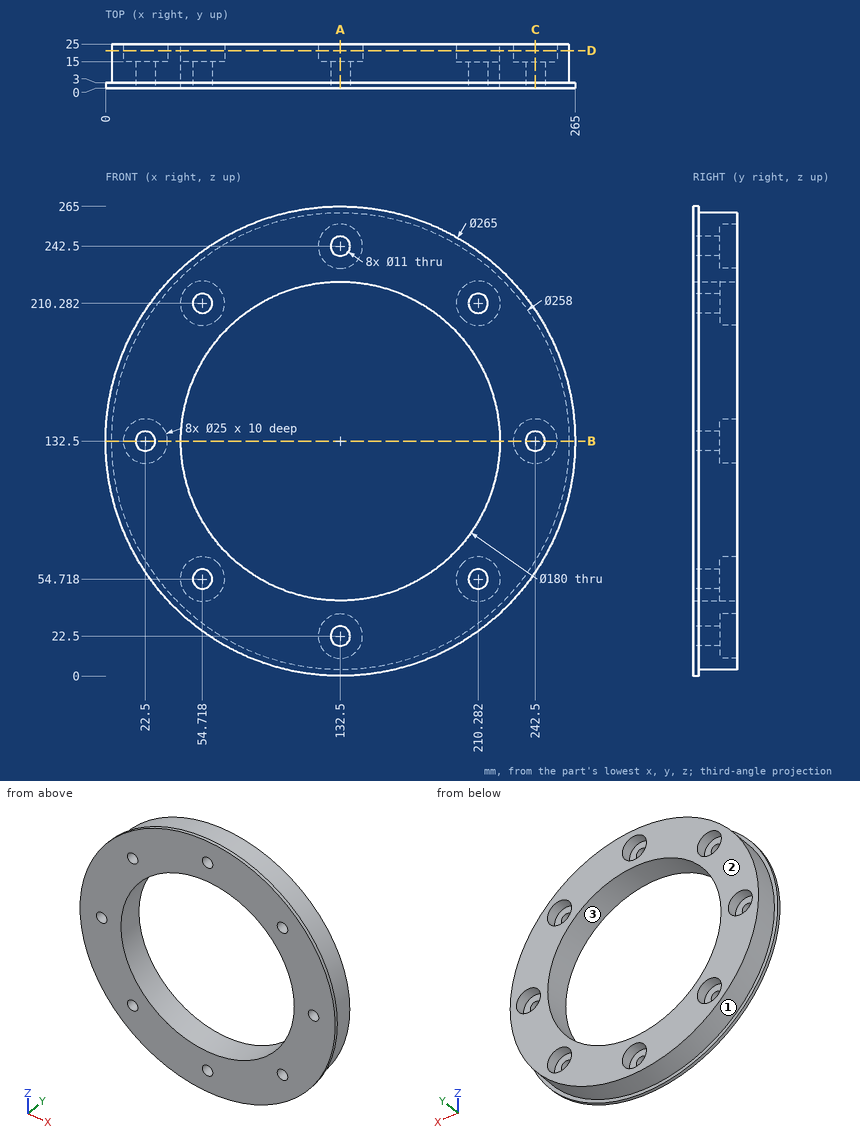
Could you check a few things on this drawing? It's one solid part, dimensions in mm from its lowest x, y, z. Round coordinates to 2 decimals unless told otherwise and drop trailing zeros. Order: outer loops, then holes, each group sorted by start corner. A loop starts at its lowest first (then second) coordinate and runs counter-clockwise, first axis right, second up.
Q1. Thinking about a two-plate mould opening in Z: for the marked faces 1, 2 and 3, which applies, released by +Z, released by -Z, zero draft, split by the parting line, or undercut?
Geometry says:
face 1: split by the parting line
face 2: zero draft
face 3: undercut
Q2. I'm going to push flat-ended pins straight in: P1, Ø1, axis at x = 152, y = 12, coming from the -Z side; P2, Ø4, axis at x = 35, y = 13.5, coming from the +Z side; P3, Ø12.5, axis at x = 210.28, z = 54.72, coming from the +Y side. Where does each tip first touch, or does it pass through?
Geometry says:
P1: stops at z = 4.91
P2: stops at z = 219.22
P3: stops at y = 15
Q3. Imagine slicing it at C-C, the plane x = 242.5. List the corners of the cut face in (y, z) for me, then the cut area to 3 significant figures.
Geometry says:
outline: (0, 58.63) - (3, 58.63) - (3, 65.11) - (25, 65.11) - (25, 120) - (15, 120) - (15, 127) - (0, 127) - close; (0, 138) - (15, 138) - (15, 145) - (25, 145) - (25, 199.89) - (3, 199.89) - (3, 206.37) - (0, 206.37) - close
area: 2,990 mm2
Q4. Imagine slicing it at A-A, the plane x = 132.5. List the corners of the cut face in (y, z) for me, then the cut area to 3 significant figures.
Geometry says:
outline: (0, 0) - (3, 0) - (3, 3.5) - (25, 3.5) - (25, 10) - (15, 10) - (15, 17) - (0, 17) - close; (0, 28) - (15, 28) - (15, 35) - (25, 35) - (25, 42.5) - (0, 42.5) - close; (0, 222.5) - (25, 222.5) - (25, 230) - (15, 230) - (15, 237) - (0, 237) - close; (0, 248) - (15, 248) - (15, 255) - (25, 255) - (25, 261.5) - (3, 261.5) - (3, 265) - (0, 265) - close
area: 1,140 mm2
Q5. Please list where these lines run through material, in increasing order: probe 1 along Z at (x, y) = (133.5, 18.75) (1 decimal); probe 2 along X at (y, z) = (13.25, 128); probe 3 along Z at (x, y) = (246, 8) (1 decimal).
Geometry says:
probe 1: z = 3.5 to 10, 35 to 42.5, 222.5 to 230, 255 to 261.5
probe 2: x = 3.58 to 19.34, 25.66 to 42.61, 222.39 to 239.34, 245.66 to 261.42
probe 3: z = 71.2 to 128.3, 136.7 to 193.8
Q6. Imagine slicing it at B-B, the plane z = 132.5. List the corners of the cut face in (x, y) for me.
Geometry says:
outline: (0, 0) - (17, 0) - (17, 15) - (10, 15) - (10, 25) - (3.5, 25) - (3.5, 3) - (0, 3) - close; (28, 0) - (42.5, 0) - (42.5, 25) - (35, 25) - (35, 15) - (28, 15) - close; (222.5, 0) - (237, 0) - (237, 15) - (230, 15) - (230, 25) - (222.5, 25) - close; (248, 0) - (265, 0) - (265, 3) - (261.5, 3) - (261.5, 25) - (255, 25) - (255, 15) - (248, 15) - close
Q7. Imagine slicing it at D-D, the plane y = 21.25. State how many separate pieces and enclosed holes the cut face has, then the cut area to 3 significant figures.
Geometry says:
separate pieces: 1
enclosed holes: 9
area: 22,900 mm2
